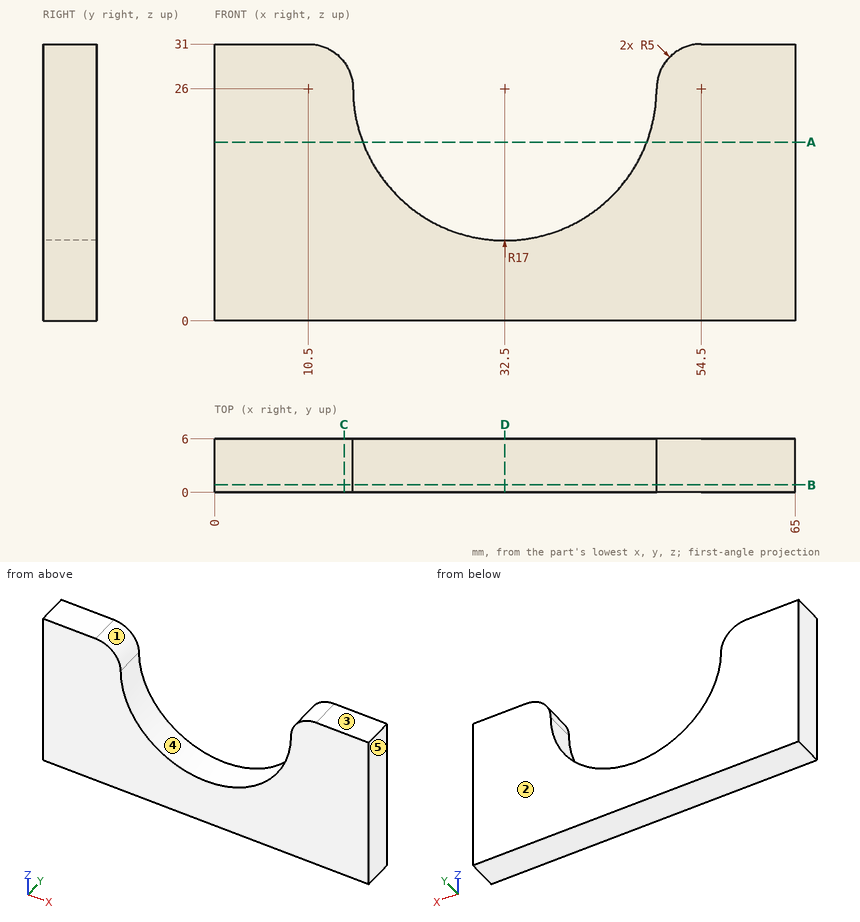
The drawing under review shows one solid part. Ordinate dimensions are in mm from its lowest x, y, z. A direction names the side the tool comes from. Round coordinates to 2 decimals unless told otherwise and drop trailing zeros. Order: outer loops, then holes, each group sorted by start corner. A loop starts at its lowest first (then second) coordinate and runs counter-clockwise, first axis right, second up. Notation, with made-up numbers: (5, -30.5) -> (9, -30.5) arc R25 cw to (9, -16.5) -> close; hole circle Ø10 at (-12, 6.25). An arc over 180 degrees is marked (long way). Use a Markdown table: item, result.
Q1. For line 1 (X direction, y = 2, z = 25.5); line 2 (X direction, y = 0.75, z = 18); line 3 (Z direction, x = 33, y = 5.3), list the stretches that pass through material, from the lowest coordinate up.
Values:
| item | result |
|---|---|
| line 1 | x = 0 to 15.51, 49.49 to 65 |
| line 2 | x = 0 to 17.5, 47.5 to 65 |
| line 3 | z = 0 to 9.01 |
Q2. Tool access review of the marked faces 1 and 2: name each direction out of +Z, -Z, +X, -X, +Y, -Y from which nothing blocks a thin tool from reaching the whole face with its end or side.
Values:
| item | result |
|---|---|
| face 1 | +Z, +Y, -Y |
| face 2 | +Z, -Z, +X, -X, +Y |
Q3. We need section D-D on x = 32.5. Write out the cut boundary in (y, z).
Values:
| item | result |
|---|---|
| outline | (0, 0) -> (6, 0) -> (6, 9) -> (0, 9) -> close |
Q4. We need section C-C on x = 14.5. Write out the cut boundary in (y, z), then the cut area to 3 significant figures.
Values:
| item | result |
|---|---|
| outline | (0, 0) -> (6, 0) -> (6, 29) -> (0, 29) -> close |
| area | 174 mm^2 |
Q5. We need section A-A on z = 20. Write out the cut boundary in (x, y).
Values:
| item | result |
|---|---|
| outline | (0, 0) -> (16.59, 0) -> (16.59, 6) -> (0, 6) -> close; (48.41, 0) -> (65, 0) -> (65, 6) -> (48.41, 6) -> close |
Q6. Clearance check with flat-ended pins moving along their axes: P1, Ø10, axis at x = 54, z = 17.5, coming from the -Y side; P2, Ø3, axis at x = 49.5, y = 5.5, coming from the +Z side; P3, Ø1, axis at x = 18, y = 4.5, coming from the +Z side. State where each tip first meets the part, or that it passes through.
Values:
| item | result |
|---|---|
| P1 | stops at y = 0 |
| P2 | stops at z = 29.57 |
| P3 | stops at z = 18 |
Q7. We need section B-B on y = 0.85. Write out the cut boundary in (x, z).
Values:
| item | result |
|---|---|
| outline | (0, 0) -> (65, 0) -> (65, 31) -> (54.5, 31) arc R5 ccw to (49.5, 26) arc R17 cw to (15.5, 26) arc R5 ccw to (10.5, 31) -> (0, 31) -> close |
Q8. Mouldability with a two-part tool opening along X and no side actions: class the marked faces 3, 4 and 5 as +X half, -X half, draft (parallel to the pull), parting line (faces both ways), or undercut.
Values:
| item | result |
|---|---|
| face 3 | draft |
| face 4 | undercut |
| face 5 | +X half |
